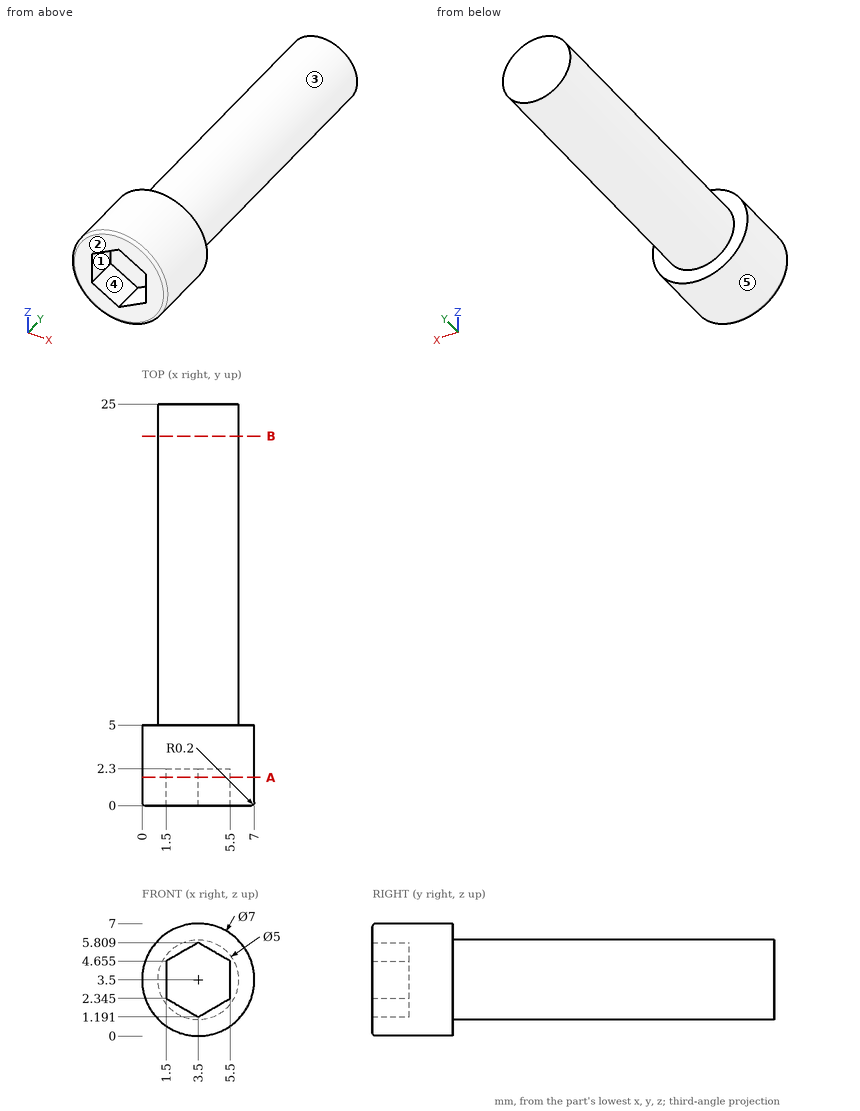
Geometry: see drawing. Coordinates: mm, zero at the bounding-box minimum. A direction names the side the tool comes from. Coordinates: 2 decimals unless noted, no trailing zeros. Order: outer loops, then holes, each group sorted by start corner. A loop starts at its lowest first (then second) coordinate and runs counter-clockwise, first axis right, second up. Notation, with made-up numbers: M 88.5,11 L 146.5,11 A12 ccw 146.5,33 Z; hole C 2,3 d7. An arc over 180 degrees is marked long. Write item = value, one per line. Start each with the question number.
(1) Line query: line 1 along Y through (x, z) = (1, 2.25); line 2 along Y through (x, z) = (2.25, 4); line 3 along X through (y, z) = (10.25, 5). Output: solid intervals per line, ascending. Write a range as [from, to].
(2) Section B-B on y = 23. Output: boundary loops of the cut face in (x, z).
(3) Section A-A on y = 1.75. Output: boundary loops of the cut face in (x, z) (1 decimal).
(4) First-contact query: P1, Ø4, axis at x = 6, y = 10, coming from the -Z side; P2, Ø4, axis at y = 8.5, z = 1, coming from the -X side. Flat tips, straight axial feed; report the tip coordinate or a pass-through.
(5) Pull-direction query (X, two-part tool) for the marked faces 1, 2 and 3; classes: released by +X, released by -X, zero draft, split by the parting line, or undercut.
(6) Reachability of the marked faces 4 and 5 from +Z, -Z, +X, -X, +Y, -Y: full face, straight path, thin tool, end or side. Return the list, or none.
Result set:
q1.line_1 = [0, 5]
q1.line_2 = [2.3, 25]
q1.line_3 = [1.5, 5.5]
q2.outline = C 3.5,3.5 d5
q3.outline = C 3.5,3.5 d7; hole M 1.5,2.3 L 3.5,1.2 L 5.5,2.3 L 5.5,4.7 L 3.5,5.8 L 1.5,4.7 Z
q4.P1 = 1.05
q4.P2 = 1.05
q5.face_1 = undercut
q5.face_2 = zero draft
q5.face_3 = split by the parting line
q6.face_4 = -Y
q6.face_5 = +Y, -Y
